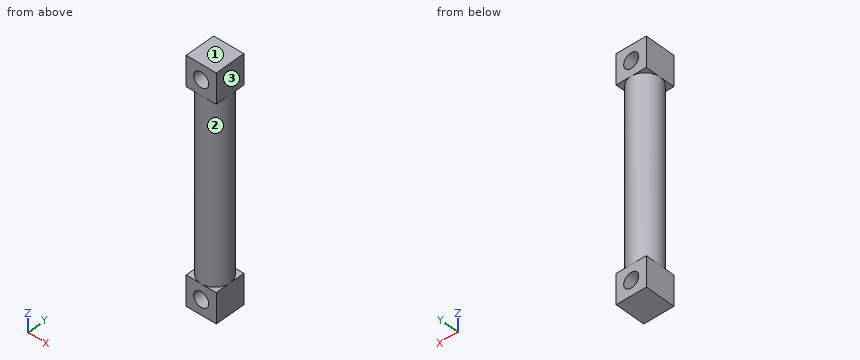
Autodesk Inventor part; units mm, degrees
ref_plane "YZ Plane" through (0, 0, 0) normal (1, 0, 0) x (0, 1, 0)
ref_plane "XZ Plane" through (0, 0, 0) normal (0, 1, 0) x (-1, 0, 0)
ref_plane "XY Plane" through (0, 0, 0) normal (0, 0, 1) x (1, 0, 0)
sketch "Sketch1" plane through (0, 0, 0) normal (0, 0, 1) x (1, 0, 0)
  circle A0 centre (0, 0) radius 6.35
  dimension "d0" = 12.7
extrude "Extrusion1" add sketch "Sketch1" along normal blind 76.2
sketch "Sketch2" plane through (0, 0, 76.2) normal (0, 0, 1) x (1, 0, 0)
  line L0 (-6.35, 6.35) -> (6.35, 6.35)
  line L1 (6.35, 6.35) -> (6.35, -6.35)
  line L2 (6.35, -6.35) -> (-6.35, -6.35)
  line L3 (-6.35, -6.35) -> (-6.35, 6.35)
extrude "Extrusion2" add sketch "Sketch2" along normal blind 12.7
sketch "Sketch3" plane through (0, 0, 0) normal (0, 0, -1) x (-1, 0, 0)
  line L0 (-6.35, 6.35) -> (6.35, 6.35)
  line L1 (6.35, 6.35) -> (6.35, -6.35)
  line L2 (6.35, -6.35) -> (-6.35, -6.35)
  line L3 (-6.35, -6.35) -> (-6.35, 6.35)
extrude "Extrusion3" add sketch "Sketch3" along normal blind 12.7
sketch "Sketch4" plane through (-6.35, -6.35, 76.2) normal (0, -1, 0) x (1, 0, 0)
  line L0 (12.7, 0) -> (12.7, 12.7)
  circle A0 centre (6.35, 6.35) radius 3.175
  circle A1 centre (6.35, -82.55) radius 3.175
  line L1 (12.7, -76.2) -> (12.7, -88.9)
  point P0 (6.35, -76.2)
  dimension "d7" = 6.35
  dimension "d8" = 6.35
  dimension "d9" = 6.35
  dimension "d10" = 6.35
  dimension "d11" = 6.35
extrude "Extrusion4" cut sketch "Sketch4" against normal blind 25.4
properties part number "3 inch piston"
Model file for the job. Use its own axes, mm. Face numbers are marked on the shaded views. Round coordinates to 2 decimals unless told otherwise and drop trailing zeros. Loops run counter-clockwise (first coordinate to the right, second up) from the corner with the lowest first, then second, coordinate; pieces in that order, holes last. Notation, with made-up numbers: (-3.5, 80) -> (51.5, 80) arc R18 ccw to (51.5, 115) -> close; hole circle Ø4 at (45.25, 87.25). An arc over 180 degrees is marked (long way). Answer as CSV lines item,"result". Start each with the question number.
1) Slice it at D-D (z = 47.5). List the corners of the cut face in (x, y).
2) Pin check, flat tips, straight feed: P1, Ø1.5, axis at x = -2, z = 7.5, coming from the -Y side; P2, Ø3, axis at x = -3.5, z = 16, coming from the -Y side; P3, Ø4, axis at x = 0, z = -6.35, coming from the -Y side; P4, Ø3, axis at x = 2, z = 20.5, coming from the +Y side. Stop position of each tip, or through.
3) Mould opens along Z. For the marked faces 1, 2 and 3 say: +Z half, -Z half, draft (parallel to the pull), parting line (faces both ways), or undercut.
4) Probe line 1 along Z through (x, y) = (0, 0.25) (3 decimals); line 2 along Z through (x, y) = (-1, 5); line 3 along Z through (x, y) = (5, -5.25). List the from-to ranges inside material, lowest first.
5) Slice it at C-C (y = -5.5). List the corners of the cut face in (x, z) (3 decimals), plus the area to 3 significant figures.
6) Slice it at A-A (z = 82.55). List the corners of the cut face in (x, y) (3 decimals), plus the area to 3 significant figures.
7) Slice it at B-B (x = 1). List the corners of the cut face in (y, z).
Filled in:
1,outline,"circle Ø12.7 at (0, 0)"
2,P1,"stops at y = -6.23"
2,P2,"stops at y = -6.03"
2,P3,"passes through"
2,P4,"stops at y = 6.33"
3,face 1,"+Z half"
3,face 2,"undercut"
3,face 3,"draft"
4,line 1,"z = -12.7 to -9.525, -3.175 to 79.375, 85.725 to 88.9"
4,line 2,"z = -12.7 to -9.36, -3.34 to 79.54, 85.56 to 88.9"
4,line 3,"z = -12.7 to 0, 76.2 to 88.9"
5,outline,"(-6.35, -12.7) -> (6.35, -12.7) -> (6.35, 0) -> (3.174, 0) -> (3.174, 76.2) -> (6.35, 76.2) -> (6.35, 88.9) -> (-6.35, 88.9) -> (-6.35, 76.2) -> (-3.174, 76.2) -> (-3.174, 0) -> (-6.35, 0) -> close; hole circle Ø6.35 at (0, -6.35); hole circle Ø6.35 at (0, 82.55)"
5,area,"743 mm2"
6,outline,"(-6.35, -6.35) -> (-3.175, -6.35) -> (-3.175, 6.35) -> (-6.35, 6.35) -> close; (3.175, -6.35) -> (6.35, -6.35) -> (6.35, 6.35) -> (3.175, 6.35) -> close"
6,area,"80.6 mm2"
7,outline,"(-6.35, -12.7) -> (6.35, -12.7) -> (6.35, -9.36) -> (-6.35, -9.36) -> close; (-6.35, -3.34) -> (6.35, -3.34) -> (6.35, 0) -> (6.27, 0) -> (6.27, 76.2) -> (6.35, 76.2) -> (6.35, 79.54) -> (-6.35, 79.54) -> (-6.35, 76.2) -> (-6.27, 76.2) -> (-6.27, 0) -> (-6.35, 0) -> close; (-6.35, 85.56) -> (6.35, 85.56) -> (6.35, 88.9) -> (-6.35, 88.9) -> close"
